from build123d import *

# Parameters (mm, degrees)
F2_R = 3
F3_R = 0.5


with BuildPart() as f1:
    # F0 (on Front) → F1 (revolve)
    with BuildSketch(Plane.XZ):
        Polygon((-17.137806, 27), (-19.5, 0), (-16.5, 0), (-16.5, 5), (-15, 5), (-15, 24), (0, 24), (0, 27), align=None)
    revolve(axis=Axis((0, 0, 19.736372), (0, 0, 1)))

    # F2
    f2_edges = [f1.edges().sort_by_distance(p)[0] for p in [
        (17.137806, 0, 27),
    ]]
    fillet(f2_edges, radius=F2_R)

    # F3
    f3_edges = [f1.edges().sort_by_distance(p)[0] for p in [
        (19.5, 0, 0),
    ]]
    fillet(f3_edges, radius=F3_R)


solid = f1.part
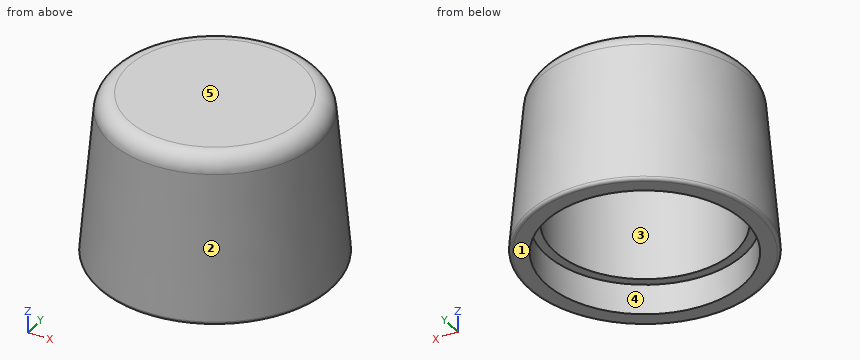
The listing builds one solid part. Answer for the finished solid, in the listing's coordinates (mm). Face numbers are marked on the shaded views. A direction names the side the tool comes from. Give positions to 0.01 mm unless a question says otherwise; leave off trailing zeros. Write each loop counter-clockwise with the first axis right and the second up, starting at its lowest first coordinate (ties: lowest second). Pieces come first, ordered by that corner, then holes. Notation, with made-up numbers: (-19.75, 31.25) -> (7.25, 31.25) arc R16 ccw to (7.25, 35.25) -> close; hole circle Ø10 at (-5, 68.5). An arc over 180 degrees is marked (long way). Use a Markdown table: item, result.
(1) Section C-C, the plane z = 16.75 is taken. Determine the outline of the cut face in (x, y).
Return value:
| item | result |
|---|---|
| outline | circle Ø36.07 at (0, 0); hole circle Ø30 at (0, 0) |
(2) Determine the mould class of the marked faces 1, 2 and 3 for opening direction Y: released by +Y, released by -Y, zero draft, split by the parting line, or undercut.
Return value:
| item | result |
|---|---|
| face 1 | zero draft |
| face 2 | split by the parting line |
| face 3 | undercut |
(3) Section A-A, the plane y = 0 is taken. Determine the outline of the cut face in (x, z).
Return value:
| item | result |
|---|---|
| outline | (-19.45, 0.54) arc R0.5 ccw to (-18.95, 0) -> (-16.5, 0) -> (-16.5, 5) -> (-15, 5) -> (-15, 24) -> (15, 24) -> (15, 5) -> (16.5, 5) -> (16.5, 0) -> (18.95, 0) arc R0.5 ccw to (19.45, 0.54) -> (17.38, 24.26) arc R3 ccw to (14.39, 27) -> (-14.39, 27) arc R3 ccw to (-17.38, 24.26) -> close |
(4) For the marked faces 4 and 5, determine the directions among +Z, -Z, +X, -X, +Y, -Y from which every point of the face is accessible in a straight line to the end or side of a thin tool.
Return value:
| item | result |
|---|---|
| face 4 | -Z |
| face 5 | +Z, +X, -X, +Y, -Y |
(5) Flat-ended cylindrical pins translate along their axes: P1, Ø9, axis at x = -0.5, y = -4, coming from the -Z side; P2, Ø1, axis at y = -2.5, z = 13.5, coming from the -X side; P3, Ø1.5, axis at x = 14, z = 4, coming from the -Y side. Find the tip coordinate at first contact, or state that the pin passes through.
Return value:
| item | result |
|---|---|
| P1 | z = 24 |
| P2 | x = -18.22 |
| P3 | y = -13.83 |
(6) Find the intervals of material crossed by probe 1 along Z at (x, y) = (10, -7); probe 2 along Y at (x, z) = (14.5, 2); probe 3 along Y at (x, z) = (11.5, 23.75), in increasing order. Write a range as from..to.
Return value:
| item | result |
|---|---|
| probe 1 | 24..27 |
| probe 2 | -12.78..-7.87, 7.87..12.78 |
| probe 3 | -13.09..-9.63, 9.63..13.09 |
